For this review, take the finished solid that the model builds, in its own axes (mm). Coordinates: 2 decimals unless noted, no trailing zeros. Write each loop counter-clockwise with the first axis right and the second up, starting at its lowest first coordinate (ties: lowest second). Pieces come first, ordered by that corner, then holes. Notation, with made-up numbers: M 49.25,16.25 L 54.25,16.25 A20 ccw 54.25,49.25 Z; hole C 78.5,47 d3. An arc over 180 degrees is marked long. Return JSON: item names as keys, results as strings.
```python
from build123d import *

# Parameters (mm, degrees)
ESQUISSE1_R             = 4.7
BOSS_EXTRU_1_DEPTH      = 5
ENL_V_START             = -10
ENL_V_MAT_EXTRU_1_DEPTH = 10
ENL_V_MAT_EXTRU_2_DEPTH = 10


with BuildPart() as part:
    # Esquisse1 → Boss.-Extru.1 (new body)
    with BuildSketch(Plane.XY):
        with BuildLine():
            Line((174.481446525, 13.461976776), (160.509166102, 40.333250621))
            Line((160.509166102, 40.333250621), (97.428399446, 20.476493551))
            Line((97.428399446, 20.476493551), (60.521806411, 91.454683092))
            Line((60.521806411, 91.454683092), (113.006926452, 131.688824037))
            Line((113.006926452, 131.688824037), (111.232668913, 135.101048724))
            ThreePointArc((111.232668913, 135.101048724), (-147.549372919, 94.096665994), (-75.582309389, -157.836353567))
            Line((-75.582309389, -157.836353567), (-45.324963396, -159.171640695))
            Line((-45.324963396, -159.171640695), (-30.981036128, -94.613715745))
            Line((-30.981036128, -94.613715745), (48.941175647, -98.140763381))
            Line((48.941175647, -98.140763381), (57.542403784, -163.71128113))
            Line((57.542403784, -163.71128113), (61.384605816, -163.880841372))
            ThreePointArc((61.384605816, -163.880841372), (147.549372919, -94.096665994), (174.481446525, 13.461976776))
        make_face()
        with Locations((121.484345953, 17.565156526)):
            Circle(ESQUISSE1_R, mode=Mode.SUBTRACT)
        with Locations((67.796167173, 55.788401035)):
            Circle(ESQUISSE1_R, mode=Mode.SUBTRACT)
        with Locations((14.416088947, -86.607403569)):
            Circle(ESQUISSE1_R, mode=Mode.SUBTRACT)
        with Locations((-45.530301203, -113.99110802)):
            Circle(ESQUISSE1_R, mode=Mode.SUBTRACT)
        with BuildLine():
            Line((-11.899961997, 30.243030676), (-20.91966999, 40.95026504))
            Line((-20.91966999, 40.95026504), (-33.702084088, 30.182438475))
            Line((-33.702084088, 30.182438475), (-32.320681925, 61.484742172))
            Line((-32.320681925, 61.484742172), (-37.315820161, 61.705182649))
            Line((-37.315820161, 61.705182649), (-42.606391614, -58.178135013))
            Line((-42.606391614, -58.178135013), (-37.611253378, -58.398575491))
            Line((-37.611253378, -58.398575491), (-35.034065472, 0))
            Line((-35.034065472, 0), (-32.5, 0))
            ThreePointArc((-32.5, 0), (-8.99280662, -31.231065129), (27.523349483, -17.283380261))
            Line((27.523349483, -17.283380261), (31.660744165, -17.465967651))
            Line((31.660744165, -17.465967651), (29.723210042, -61.370113123))
            Line((29.723210042, -61.370113123), (34.718348278, -61.590553601))
            Line((34.718348278, -61.590553601), (40.008919731, 58.292764062))
            Line((40.008919731, 58.292764062), (35.013781495, 58.513204539))
            Line((35.013781495, 58.513204539), (33.203827505, 17.5))
            Line((33.203827505, 17.5), (27.21544776, 17.764273225))
            ThreePointArc((27.21544776, 17.764273225), (9.877796967, 30.962543937), (-11.899961997, 30.243030676))
        make_face(mode=Mode.SUBTRACT)
    extrude(amount=BOSS_EXTRU_1_DEPTH)

    # Esquisse2 → Enlèv. mat.-Extru.1 (cut)
    with BuildSketch(Plane.XY.offset(5).offset(ENL_V_START)):
        with BuildLine():
            Line((-88.148964429, 43.929034477), (-152.860619324, 85.197600084))
            ThreePointArc((-152.860619324, 85.197600084), (-174.829838257, 7.715416702), (-159.771465705, -71.400831554))
            Line((-159.771465705, -71.400831554), (-91.676012064, -35.993177298))
            Line((-91.676012064, -35.993177298), (-88.148964429, 43.929034477))
        make_face()
    extrude(amount=ENL_V_MAT_EXTRU_1_DEPTH, mode=Mode.SUBTRACT)

    # Esquisse3 → Enlèv. mat.-Extru.2 (cut)
    with BuildSketch(Plane.XY.offset(5)):
        Polygon((40.948954466, -97.788058617), (-12.998538482, -95.407301464), (-12.116776573, -75.42674852), (41.830716375, -77.807505674), align=None)
        Polygon((-49.436008781, -85.46488415), (-29.912121681, -89.802836721), (-41.624593625, -142.517331891), (-61.148480724, -138.179379319), align=None)
        Polygon((64.212465714, 84.356864138), (89.124416013, 36.446586197), (71.379868627, 27.219937939), (46.467918329, 75.130215879), align=None)
        Polygon((98.732765194, -0.080397389), (92.727598771, 18.996761106), (144.235926707, 35.210710447), (150.24109313, 16.133551952), align=None)
    extrude(amount=-ENL_V_MAT_EXTRU_2_DEPTH, mode=Mode.SUBTRACT)


solid = part.part
```
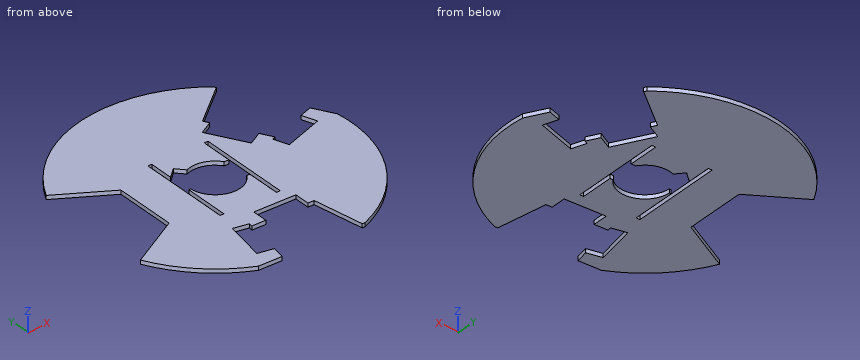
1. We need section C-C (y = -130). State the section outline as (x, z) points.
Checks:
{"outline": "M -117.15,0 L -59.33,0 L -59.33,5 L -117.15,5 Z; M 53.12,0 L 117.15,0 L 117.15,5 L 53.12,5 Z"}
2. Clearance check with flat-ended pins moving along their axes: pin 1 Ø0.8 at (x, z) = (-33.5, 3.5) entering from +Y; pin 2 Ø1 at (y, z) = (-110.5, 2) entering from -X; pin 3 Ø3 at (x, z) = (-89.5, 1) entering from +Y. State where each tip first meets the part, or that it passes through.
Checks:
{"pin 1": "y = 171.84", "pin 2": "x = -136.11", "pin 3": "y = 151.26"}
3. We need section B-B (y = -49.5). State the section outline as (x, z) points, plus the area to 3 significant figures.
Checks:
{"outline": "M -117.65,0 L -42.22,0 L -42.22,5 L -117.65,5 Z; M -37.22,0 L 30.25,0 L 30.25,5 L -37.22,5 Z; M 35.25,0 L 167.85,0 L 167.85,5 L 35.25,5 Z", "area": "1,380 mm2"}
4. We need section A-A (x = -4). State the section outline as (y, z) points.
Checks:
{"outline": "M -75.78,0 L -32.25,0 L -32.25,5 L -75.78,5 Z; M 32.25,0 L 174.95,0 L 174.95,5 L 32.25,5 Z"}
5. We need section D-D (y = 8). State the section outline as (x, z) points, plus the area to 3 significant figures.
Checks:
{"outline": "M -89.73,0 L -39.69,0 L -39.69,5 L -89.73,5 Z; M 37.79,0 L 96.19,0 L 96.19,5 L 37.79,5 Z; M 124.4,0 L 174.82,0 L 174.82,5 L 124.4,5 Z", "area": "794 mm2"}
6. Wall thickness on L1, parallel to X at y = 29, z = 1.4; L2, parallel to X at y = 43, z = 4.5; L3, parallel to X at y = -49.5, z = 2.3: over which ranges is each line inside the solid? List them lowest first. Write a range as from..to.
Checks:
{"L1": "-88.81..-38.76, 14.67..33.71, 38.72..70.45, 74.8..93, 146.19..166.4", "L2": "-88.19..-38.14, -33.14..34.33, 39.33..63.17", "L3": "-117.65..-42.22, -37.22..30.25, 35.25..167.85"}
